Verification items for the finished model (mm, model axes). A direction names the side the tool comes from. Give positions to 0.01 mm unless a question says otherwise; leave off trailing zeros. Loops run counter-clockwise (first coordinate to the right, second up) from the corner with the lowest first, then second, coordinate; pieces in that order, holes last. Notation, with made-up numbers: (-6.75, 77.25) - (50.25, 77.25) arc R21 cw to (50.25, 105.25) - close; hole circle Ø7 at (49, 41). An arc over 180 degrees is marked (long way). Answer in a Markdown table with one row per item.
```python
from build123d import *

# Parameters (mm, degrees)
F1_DEPTH = 25.4
F2_W     = 12.7
F2_H     = 12.7
F3_DEPTH = 25.4
F4_W     = 6.35
F4_H     = 12.7
F5_DEPTH = 12.7


with BuildPart() as f1:
    # F0 (on Top) → F1 (new body)
    with BuildSketch(Plane.XY):
        Polygon((25.4, -12.7), (25.4, 12.7), (0, 12.7), (-25.4, 12.7), (-25.4, -12.7), (-25.4, -38.1), (0, -38.1), (0, -12.7), align=None)
    extrude(amount=F1_DEPTH)

    # F2 (on face) → F3 (join)
    with BuildSketch(Plane.XY.offset(25.4)):
        with Locations((-10.5918, -2.1082)):
            Rectangle(F2_W, F2_H)
    extrude(amount=F3_DEPTH)

    # F4 (on face) → F5 (cut)
    with BuildSketch(Plane.XY.offset(50.8)):
        with Locations((-7.4168, -2.1082)):
            Rectangle(F4_W, F4_H)
    extrude(amount=-F5_DEPTH, mode=Mode.SUBTRACT)


solid = f1.part
```
Q1. Tool access check on faces 1 (the face through (13, -12.7, 13)), 2 (the face through (-10.592, -2, 45)), 3 (the face through (-16.942, -2, 38)), 4 (the face through (-12, 4.242, 35)). Record the directions out of +Z, -Z, +X, -X, +Y, -Y that give a thin tool (end or side, any length) a straight path to the whole face; none if there is none.
Completed:
| item | result |
|---|---|
| face 1 | +Z, -Z, +X, -Y |
| face 2 | +Z, +X, +Y, -Y |
| face 3 | +Z, -X, +Y, -Y |
| face 4 | +Z, +X, -X, +Y |
Q2. Sectioned sample at A-A (y = 0.5). Record the cut outline in (x, z).
Completed:
| item | result |
|---|---|
| outline | (-25.4, 0) - (25.4, 0) - (25.4, 25.4) - (-4.24, 25.4) - (-4.24, 38.1) - (-10.59, 38.1) - (-10.59, 50.8) - (-16.94, 50.8) - (-16.94, 25.4) - (-25.4, 25.4) - close |
Q3. Thickness scan on line 1 (Y direction, x = 0.5, z = 23.5); line 2 (Y direction, x = -15, z = 46); line 3 (Z direction, x = 5.5, y = 4.5). Record the ranges inside material, lowest first.
Completed:
| item | result |
|---|---|
| line 1 | -12.7 to 12.7 |
| line 2 | -8.46 to 4.24 |
| line 3 | 0 to 25.4 |
Q4. Sectioned sample at C-C (x = 6.5). Record the cut outline in (y, z).
Completed:
| item | result |
|---|---|
| outline | (-12.7, 0) - (12.7, 0) - (12.7, 25.4) - (-12.7, 25.4) - close |
Q5. Sectioned sample at B-B (z = 15). Record the cut outline in (x, y), and give its area (3 significant figures).
Completed:
| item | result |
|---|---|
| outline | (-25.4, -38.1) - (0, -38.1) - (0, -12.7) - (25.4, -12.7) - (25.4, 12.7) - (-25.4, 12.7) - close |
| area | 1,940 mm^2 |
Q6. Go/stop test with flat-tipped pins: P1, Ø12.5, axis at x = 7.5, z = 19, coming from the -Y side; P2, Ø6, axis at x = -0.5, z = 35, coming from the +Y side; P3, Ø12, axis at x = -4.5, y = -26.5, coming from the -Z side; P4, Ø10, axis at y = -5, z = 33, coming from the +X side. Record where each tip stops, or that it passes through.
Completed:
| item | result |
|---|---|
| P1 | y = -12.7 |
| P2 | through |
| P3 | z = 0 |
| P4 | x = -4.24 |
Q7. Sectioned sample at D-D (z = 29). Record the cut outline in (x, y).
Completed:
| item | result |
|---|---|
| outline | (-16.94, -8.46) - (-4.24, -8.46) - (-4.24, 4.24) - (-16.94, 4.24) - close |
